Part model, mm, in its own coordinate system. A direction names the side the tool comes from. Round coordinates to 2 decimals unless told otherwise and drop trailing zeros. Loops run counter-clockwise (first coordinate to the right, second up) from the corner with the lowest first, then second, coordinate; pieces in that order, holes last. Notation, with made-up numbers: M -11.5,-14 L 14.5,-14 A32 cw 14.5,19 Z; hole C -33,-39.75 d9. An arc over 180 degrees is marked long. Put each result on its own line as item: value. Start each with the question number.
1) Slice it at B-B on x = -13.75. Give the cut face in (y, z).
2) Probe line 1 along Z through (x, y) = (-16, 2.8); line 2 along X through (y, z) = (1.35, -23); line 3 along Z through (x, y) = (25.5, -0.55). List the from-to ranges inside material, lowest first.
3) Slice it at A-A on z = 0. Give the cut face in (x, y), then the cut area to 3 significant figures.
4) Pull direction Z, two halves, no side cores. Call faces 3 (the cylindrical face through (-22.818, 0.535, -29.759)), 4 (the flat face through (1, 3, 8)), 5 (the flat face through (0, 0, 0)): +Z half, -Z half, draft (parallel to the pull), parting line (faces both ways), or undercut.
5) Drop flat-ended pins along their axis: pin 1 Ø2.5 at (x, z) = (0, -0.5) entering from +Y; pin 2 Ø2 at (x, y) = (-7.5, -0.5) entering from +Z; pin 3 Ø3 at (y, z) = (-1, 11) entering from +X; pin 4 Ø5.5 at (x, z) = (-13.75, 23.82) entering from -Y. Give the stop position or say it passes through.
6) Which spindle directions (+Z, -Z, +X, -X, +Y, -Y) get a long thin tool onto all of the face, cutting with end or side? Do faces 1 (the cylindrical face through (0.71, 1.48, 2.24)), 2 (the cylindrical face through (-10.531, 0.535, -27.326)). Say none if no direction does.
7) Slice it at D-D on y = 1.5. State how many separate pieces and enclosed holes the cut face has, then the cut area to 3 significant figures.
8) Slice it at C-C on x = 0. Give the cut face in (y, z), then the cut area to 3 significant figures.
```python
from build123d import *

# Parameters (mm, degrees)
SKETCH1_R           = 37.5
SKETCH1_R_2         = 2.35
BOSS_EXTRUDE1_DEPTH = 3
SKETCH1_3_R         = 37.5
SKETCH1_3_R_2       = 2.35
BOSS_EXTRUDE2_DEPTH = 2
SKETCH2_R           = 4.7625
CUT_EXTRUDE1_DEPTH  = 54.268189382
CIRPATTERN1_COUNT   = 3


with BuildPart() as part:
    # Sketch1 → Boss-Extrude1 (new body)
    with BuildSketch(Plane(origin=(0, 0, 0), x_dir=(1, 0, 0), z_dir=(0, 1, 0))):
        with Locations(Location((0, 0, 0), (0, 0, 270))):
            Circle(SKETCH1_R)
        with Locations(Location((0, 0, 0), (0, 0, 270))):
            Circle(SKETCH1_R_2, mode=Mode.SUBTRACT)
    extrude(amount=BOSS_EXTRUDE1_DEPTH)

    # Sketch1_3 → Boss-Extrude2 (add)
    with BuildSketch(Plane(origin=(0, 0, 0), x_dir=(1, 0, 0), z_dir=(0, 1, 0))):
        with Locations(Location((0, 0, 0), (0, 0, 270))):
            Circle(SKETCH1_3_R)
        with Locations(Location((0, 0, 0), (0, 0, 270))):
            Circle(SKETCH1_3_R_2, mode=Mode.SUBTRACT)
        with Locations(Location((0, 0, 0), (0, 0, 270))):
            Circle(SKETCH1_3_R_2)
    extrude(amount=-BOSS_EXTRUDE2_DEPTH)

    # Sketch2 → Cut-Extrude1 (cut, through all)
    with BuildSketch(Plane(origin=(0, 3, 0), x_dir=(1, 0, 0), z_dir=(0, 1, 0))):
        with Locations(Location((27.5, 0, 0), (0, 0, 270))):
            Circle(SKETCH2_R)
    cut_extrude1 = extrude(amount=-CUT_EXTRUDE1_DEPTH, mode=Mode.SUBTRACT)

    # CirPattern1: Cut-Extrude1 ×3 about axis
    cirpattern1_axis = Axis((0, 0, 0), (0, 1, 0))
    for i in range(1, CIRPATTERN1_COUNT):
        add(cut_extrude1.rotate(cirpattern1_axis, i * 360 / CIRPATTERN1_COUNT), mode=Mode.SUBTRACT)


solid = part.part
```
Recorded:
1. outline: M -2,-34.89 L 3,-34.89 L 3,-28.58 L -2,-28.58 Z; M -2,-19.05 L 3,-19.05 L 3,19.05 L -2,19.05 Z; M -2,28.58 L 3,28.58 L 3,34.89 L -2,34.89 Z
2. line 1: z = -33.92 to -28.01, -19.62 to 19.62, 28.01 to 33.92
2. line 2: x = -29.62 to -18.44, -9.06 to 29.62
2. line 3: z = -27.5 to -4.32, 4.32 to 27.5
3. outline: M -37.5,-2 L 22.74,-2 L 22.74,3 L 2.35,3 L 2.35,0 L -2.35,0 L -2.35,3 L -37.5,3 Z; M 32.26,-2 L 37.5,-2 L 37.5,3 L 32.26,3 Z
3. area: 313 mm2
4. face 3: parting line
4. face 4: draft
4. face 5: undercut
5. pin 1: stops at y = 0
5. pin 2: stops at z = 36.93
5. pin 3: stops at x = 36.28
5. pin 4: passes through
6. face 1: +Y
6. face 2: +Y, -Y
7. separate pieces: 1
7. enclosed holes: 4
7. area: 4,190 mm2
8. outline: M -2,-37.5 L 3,-37.5 L 3,-2.35 L 0,-2.35 L 0,2.35 L 3,2.35 L 3,37.5 L -2,37.5 Z
8. area: 361 mm2
